from build123d import *

# Parameters (mm, degrees)
F0_W     = 20
F0_H     = 20
F1_DEPTH = 20
F3_W     = 20
F3_H     = 20
F3_H_2   = 5
F4_DEPTH = 5
F5_DEPTH = 20
F2_W     = 20
F2_H     = 5
F6_DEPTH = 5


with BuildPart() as f1:
    # F0 (on Right) → F1 (new body)
    with BuildSketch(Plane.YZ):
        with Locations((10, 10)):
            Rectangle(F0_W, F0_H)
    extrude(amount=-F1_DEPTH)

    # F3 (on face) → F4 (join)
    with BuildSketch(Plane(origin=(-20, 0, 0), x_dir=(0, -1, 0), z_dir=(-1, 0, 0))):
        with Locations((-10, 10)):
            Rectangle(F3_W, F3_H)
        with Locations((-10, 22.5)):
            Rectangle(F3_W, F3_H_2)
    extrude(amount=F4_DEPTH)

    # F2 (on face) → F5 (cut)
    with BuildSketch(Plane.YZ):
        Polygon((0, 5), (20, 20), (0, 20), align=None)
    extrude(amount=-F5_DEPTH, mode=Mode.SUBTRACT)

    # F2 (on face) → F6 (join)
    with BuildSketch(Plane.YZ):
        with Locations((10, 22.5)):
            Rectangle(F2_W, F2_H)
        Polygon((0, 5), (20, 20), (0, 20), align=None)
        Polygon((0, 0), (20, 0), (20, 20), (0, 5), align=None)
    extrude(amount=F6_DEPTH)


solid = f1.part
The listing builds one solid part. Answer for the finished solid, in the listing's coordinates (mm). A direction names the side the tool comes from. Coordinates: 2 decimals unless noted, no trailing zeros. Loops run counter-clockwise (first coordinate to the right, second up) from the corner with the lowest first, then second, coordinate; pieces in that order, holes last. Notation, with made-up numbers: (-28.75, -36.75) -> (29.25, -36.75) arc R14 cw to (29.25, -23.75) -> close; hole circle Ø5 at (12.25, 66). An arc over 180 degrees is marked (long way). Write item = value, one per line. Start each with the question number.
1) A tool of negligible diameter and unlimited length cuts with its end or side. For faces 1 (the face through (-20, 8, 17)), 2 (the face through (-25, 10, 13)), from which of +Z, -Z, +X, -X, +Y, -Y can it reach the whole face along a straight path? Write none if from no direction.
2) A cutting plane is placed at D-D (x = -1.25). Give the vertices of the cut face in (y, z), then the cut area to 3 significant figures.
3) A cutting plane is placed at C-C (z = 10.25). Give the vertices of the cut face in (x, y).
4) Given pin 1 Ø3 at (x, z) = (-4.5, 9) entering from -Y, flat-ended and moving along its own axis, determine where the tip first touches the part or whether it passes through.
5) A cutting plane is placed at A-A (z = 23.5). Give the vertices of the cut face in (x, y).
6) A cutting plane is placed at B-B (y = 15). Give the vertices of the cut face in (x, z), then the cut area to 3 significant figures.
7) Straight lines are drawn through the part: line 1 (X direction, y = 12, z = 16.5); line 2 (Y direction, x = -14, z = 8.5); line 3 (Z direction, x = -2, y = 11.5) (3 decimals). For each, find the intervals that lie inside material, in ascending order. Write a range as from..to.
8) The mould has two halves that part along X. Classify faces 3 (the face through (5, 10, 13)), 4 (the face through (2, 10, 25)), 5 (the face through (0, 8, 17)), 6 (the face through (-9.86, 9.86, 12.395)): released by +X, released by -X, zero draft, split by the parting line, or undercut.
Responses:
q1.face_1 = +Z, -Y
q1.face_2 = +Z, -Z, -X, +Y, -Y
q2.outline = (0, 0) -> (20, 0) -> (20, 20) -> (0, 5) -> close
q2.area = 250 mm²
q3.outline = (-25, 0) -> (-20, 0) -> (-20, 7) -> (0, 7) -> (0, 0) -> (5, 0) -> (5, 20) -> (-25, 20) -> close
q4.pin_1 = 3.33
q5.outline = (-25, 0) -> (-20, 0) -> (-20, 20) -> (-25, 20) -> close; (0, 0) -> (5, 0) -> (5, 20) -> (0, 20) -> close
q6.outline = (-25, 0) -> (5, 0) -> (5, 25) -> (0, 25) -> (0, 16.25) -> (-20, 16.25) -> (-20, 25) -> (-25, 25) -> close
q6.area = 575 mm²
q7.line_1 = -25..-20, 0..5
q7.line_2 = 4.67..20
q7.line_3 = 0..13.625
q8.face_3 = released by +X
q8.face_4 = zero draft
q8.face_5 = undercut
q8.face_6 = undercut
